```python
from build123d import *

# Parameters (mm, degrees)
F1_DEPTH     = 12.7
F0_W         = 2.54
F0_H         = 38.1
F2_DEPTH     = 12.7
F4_D         = 1.27
F5_W         = 3.81
F5_H         = 12.7
F6_DEPTH     = 6.35
F8_D         = 2.54
F9_W         = 3.81
F9_H         = 12.7
F10_DEPTH    = 6.35
F12_D        = 2.54
F12_DEPTH    = 22.86
F12_TIP      = 0.7630929862
F13_T1_DEPTH = 90.7253227153
F13_T3_DEPTH = 85.6453227153
F14_T1_DEPTH = 70.3362845074
F14_T3_DEPTH = 82.312532111
F15_T1_DEPTH = 94.0409858467
F15_T3_DEPTH = 99.4843801619


# Not quite as in the source:
# - a fillet or chamfer that OpenCascade refuses, or shapes differently, is made with other operations: its cross-section is extruded or revolved along the edge and cut away or added


with BuildPart() as f1:
    # F0 (on Top) → F1 (new body)
    with BuildSketch(Plane.XY):
        with BuildLine():
            ThreePointArc((-63.5, 0), (0, 19.05), (63.5, 0))
            Line((63.5, 0), (63.5, 38.1))
            Line((63.5, 38.1), (38.1, 38.1))
            Line((38.1, 38.1), (38.1, 54.61))
            Line((38.1, 54.61), (-38.1, 54.61))
            Line((-38.1, 54.61), (-38.1, 31.75))
            Line((-38.1, 31.75), (-69.85, 31.75))
            Line((-69.85, 31.75), (-63.5, 0))
        make_face()
    extrude(amount=F1_DEPTH)

    # F0 (on Top) → F2 (join, symmetric)
    with BuildSketch(Plane.XY):
        Polygon((-65.9142452177, -0.6287739113), (-63.5, 0), (-69.85, 31.75), (-72.39, 31.75), align=None)
        with Locations((64.77, 19.05)):
            Rectangle(F0_W, F0_H)
    extrude(amount=F2_DEPTH, both=True)

    # F4 (through all)
    with Locations(Plane.XY.offset(12.7)):
        with Locations((-45.604262501, 25.4304688424), (-54.9195222557, 25.4304688424), (-63.5848790407, 25.4304688424)):
            Hole(F4_D / 2)

    # F5 (on face) → F6 (join)
    with BuildSketch(Plane(origin=(0, 54.61, 0), x_dir=(-1, 0, 0), z_dir=(0, 1, 0))):
        with Locations((-33.655, 6.35)):
            Rectangle(F5_W, F5_H)
        with Locations((-17.145, 6.35)):
            Rectangle(F5_W, F5_H)
        with Locations((-8.255, 6.35)):
            Rectangle(F5_W, F5_H)
        with Locations((8.255, 6.35)):
            Rectangle(F5_W, F5_H)
        with Locations((17.145, 6.35)):
            Rectangle(F5_W, F5_H)
        with Locations((33.655, 6.35)):
            Rectangle(F5_W, F5_H)
    extrude(amount=F6_DEPTH)

    # F8 (through all)
    with Locations(Plane.YZ.offset(35.56)):
        with Locations((57.785, 6.35)):
            Hole(F8_D / 2)

    # F9 (on face) → F10 (join)
    with BuildSketch(Plane(origin=(0, 38.1, 0), x_dir=(-1, 0, 0), z_dir=(0, 1, 0))):
        with Locations((-45.085, 6.35)):
            Rectangle(F9_W, F9_H)
        with Locations((-61.595, 6.35)):
            Rectangle(F9_W, F9_H)
    extrude(amount=F10_DEPTH)

    # F12
    with Locations(Plane.YZ.offset(63.5)):
        with Locations((41.275, 6.35)):
            Hole(F12_D / 2, depth=F12_DEPTH)
            with Locations((0, 0, -(F12_DEPTH + F12_TIP / 2))):  # 118° drill point
                Cone(0, F12_D / 2, F12_TIP, mode=Mode.SUBTRACT)

    # F13: chamfer of 5.08 x 10.16 on 2 edges, made by hand

    # F13_s2 → F13_t1 (cut)
    with BuildSketch(Plane.XZ.offset(-64.4126613577)):
        Polygon((60.96, 12.7), (66.04, 2.54), (66.04, 12.7), align=None)
    extrude(amount=F13_T1_DEPTH, mode=Mode.SUBTRACT)

    # F13_s4 → F13_t3 (cut)
    with BuildSketch(Plane(origin=(-14.0503374507, 70.2516872533, 0), x_dir=(0, 0, 1), z_dir=(0.1961161351, -0.9805806757, 0))):
        Polygon((12.7, 59.6775478226), (2.54, 64.7575478226), (12.7, 64.7575478226), align=None)
    extrude(amount=F13_T3_DEPTH, mode=Mode.SUBTRACT)

    # F14: chamfer of 5.08 x 7.62 on 2 edges, made by hand

    # F14_s2 → F14_t1 (cut)
    with BuildSketch(Plane(origin=(-12.5630602506, 62.8153012532, 0), x_dir=(0, 0, 1), z_dir=(0.1961161351, -0.9805806757, 0))):
        Polygon((5.8844648046, 63.0853154203), (12.7, 54.5975478226), (12.7, 59.6775478226), align=None)
    extrude(amount=F14_T1_DEPTH, mode=Mode.SUBTRACT)

    # F14_s4 → F14_t3 (cut)
    with BuildSketch(Plane.XZ.offset(-64.1950058926)):
        Polygon((55.88, 12.7), (64.3677675977, 5.8844648046), (60.96, 12.7), align=None)
    extrude(amount=F14_T3_DEPTH, mode=Mode.SUBTRACT)

    # F15: chamfer of 12.7 x 5.08 on 2 edges, made by hand

    # F15_s2 → F15_t1 (cut)
    with BuildSketch(Plane(origin=(-14.9629972051, 74.8149860255, 0), x_dir=(0, 0, 1), z_dir=(0.1961161351, -0.9805806757, 0))):
        Polygon((12.7, 41.8975478226), (9.5193490439, 58.5585905509), (12.7, 54.5975478226), align=None)
    extrude(amount=F15_T1_DEPTH, mode=Mode.SUBTRACT)

    # F15_s4 → F15_t3 (cut)
    with BuildSketch(Plane.XZ.offset(-71.0983312548)):
        Polygon((59.8410427283, 9.5193490439), (43.18, 12.7), (55.88, 12.7), align=None)
    extrude(amount=F15_T3_DEPTH, mode=Mode.SUBTRACT)


solid = f1.part
```
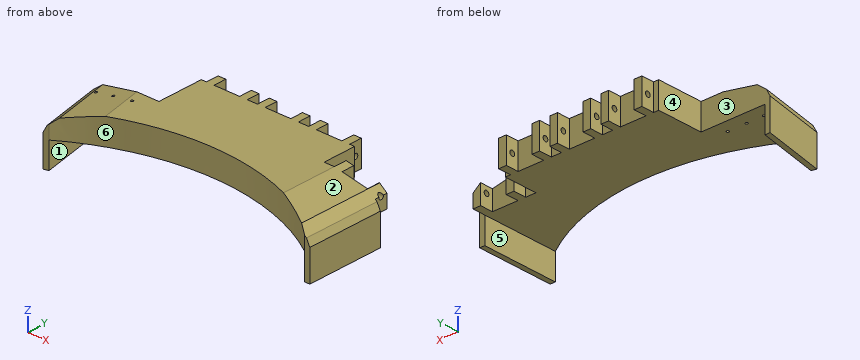
CAD build for the part. Positions are in the model's coordinates, mm. Face numbers are marked on the shaded views. A direction names the side the tool comes from. Give positions to 0.01 mm unless a question says otherwise; leave off trailing zeros. Order: outer loops, then holes, each group sorted by start corner. A loop starts at its lowest first (then second) coordinate and runs counter-clockwise, first axis right, second up. Notation, with made-up numbers: M 51.25,55 L 97.25,55 A23 ccw 97.25,64 Z; hole C 50,75.5 d5. An arc over 180 degrees is marked long. Put each result on its own line as item: value. Start each with the question number.
(1) Which spindle directions (+Z, -Z, +X, -X, +Y, -Y) get a long thin tool onto all of the face, cutting with end or side? Do the marked faces 1 and 2. Say none if no direction does.
(2) Flat gauge pins, fed straight in: pin 1 Ø6.5 at (x, z) = (-26.5, 8) entering from +Y; pin 2 Ø6 at (x, z) = (34.5, -4.5) entering from -Y; pin 3 Ø8 at (x, y) = (51.5, 25) entering from +Z; pin 4 Ø8 at (x, y) = (48, 5.5) entering from +Z. Where does each tip first touch, or does it go through?
(3) Saw through at C-C, the plane x = 8.5. Write the cut outline in (y, z) (3 decimals).
(4) Saw through at A-A, the plane z = -8.5. Write the cut outline in (x, y).
(5) Saw through at D-D, the plane x = 45. Write the cut outline in (y, z) (3 decimals), then the cut area to 3 significant figures.
(6) Saw through at B-B, the plane y = 7. Write the cut outline in (x, z).
(7) Mould opens along X. For the marked faces 3, 4, 5 and 6 say: +X half, -X half, draft (parallel to the pull), parting line (faces both ways), or undercut.
(8) Drill centre lines: line 1 along Z through (x, y) = (-37.5, 27); line 2 along X through (y, z) = (28, -11.25); line 3 along X through (y, z) = (30, -0.25). Where is each one in solid material? Low to high.
Check result:
1. face 1: -Z, +Y
1. face 2: +Z, +X, +Y, -Y
2. pin 1: stops at y = 54.61
2. pin 2: passes through
2. pin 3: stops at z = 11.88
2. pin 4: stops at z = 12.05
3. outline: M 18.736,0 L 60.96,0 L 60.96,12.7 L 18.736,12.7 Z; hole C 57.785,6.35 d2.54
4. outline: M -72.39,31.75 L -65.91,-0.63 L -63.5,0 L -69.85,31.75 Z; M 63.5,0 L 66.04,0 L 66.04,38.1 L 63.5,38.1 Z
5. outline: M 9.911,0 L 44.45,0 L 44.45,12.353 L 9.911,12.353 Z; hole C 41.275,6.35 d2.54
5. area: 422 mm2
6. outline: M -67.44,-12.7 L -64.9,-12.7 L -64.9,0 L -51.33,0 L -51.33,11.35 L -61.12,9.52 L -65.73,5.88 L -67.44,2.54 Z; M 51.33,0 L 63.5,0 L 63.5,-12.7 L 66.04,-12.7 L 66.04,2.54 L 64.37,5.88 L 59.84,9.52 L 51.33,11.14 Z
7. face 3: draft
7. face 4: -X half
7. face 5: undercut
7. face 6: undercut
8. line 1: z = 0 to 12.7
8. line 2: x = -71.64 to -69.1, 63.5 to 66.04
8. line 3: x = -72.04 to -69.5, 63.5 to 66.04
